Model file for the job. Use its own axes, mm. Face numbers are marked on the shaded views. Round coordinates to 2 decimals unless told otherwise and drop trailing zeros. Write each loop counter-clockwise with the first axis right and the second up, starting at its lowest first coordinate (ties: lowest second). Pieces come first, ordered by that corner, then holes.
```python
from build123d import *

# Parameters (mm, degrees)
BOSS_EXTRUDE1_DEPTH     = 14
SKETCH2_R               = 5
CUT_EXTRUDE1_DEPTH      = 50
SKETCH5_R               = 5
CUT_EXTRUDE3_DEPTH      = 50
CUT_EXTRUDE3_DEPTH_BACK = 50
SKETCH6_R               = 5
CUT_EXTRUDE4_DEPTH      = 50
CUT_EXTRUDE4_DEPTH_BACK = 50


with BuildPart() as part:
    # Sketch1 → Boss-Extrude1 (new body)
    with BuildSketch(Plane.XY):
        Polygon((-42.857142857, 0), (82.142857143, 0), (19.642857143, 108.253175473), align=None)
    extrude(amount=BOSS_EXTRUDE1_DEPTH)

    # Sketch2 → Cut-Extrude1 (cut)
    with BuildSketch(Plane(origin=(0, 0, 0), x_dir=(0, 0, -1), z_dir=(1, 0, 0))):
        with Locations((-7, 101.253175473)):
            Circle(SKETCH2_R)
    extrude(amount=CUT_EXTRUDE1_DEPTH, mode=Mode.SUBTRACT)

    # Sketch5 → Cut-Extrude3 (cut, two sides)
    with BuildSketch(Plane(origin=(-10.714285714, 18.557687224, 0), x_dir=(-0.866025404, -0.5, 0), z_dir=(0.5, -0.866025404, 0))) as cut_extrude3_sk:
        with Locations((30.115374448, -7)):
            Circle(SKETCH5_R)
    extrude(amount=CUT_EXTRUDE3_DEPTH, mode=Mode.SUBTRACT)
    extrude(cut_extrude3_sk.sketch, amount=-CUT_EXTRUDE3_DEPTH_BACK, mode=Mode.SUBTRACT)

    # Sketch6 → Cut-Extrude4 (cut, two sides)
    with BuildSketch(Plane(origin=(20.535714286, 35.568900513, 0), x_dir=(0.866025404, -0.5, 0), z_dir=(0.5, 0.866025404, 0))) as cut_extrude4_sk:
        with Locations((64.137801025, -7)):
            Circle(SKETCH6_R)
    extrude(amount=CUT_EXTRUDE4_DEPTH, mode=Mode.SUBTRACT)
    extrude(cut_extrude4_sk.sketch, amount=-CUT_EXTRUDE4_DEPTH_BACK, mode=Mode.SUBTRACT)


solid = part.part
```
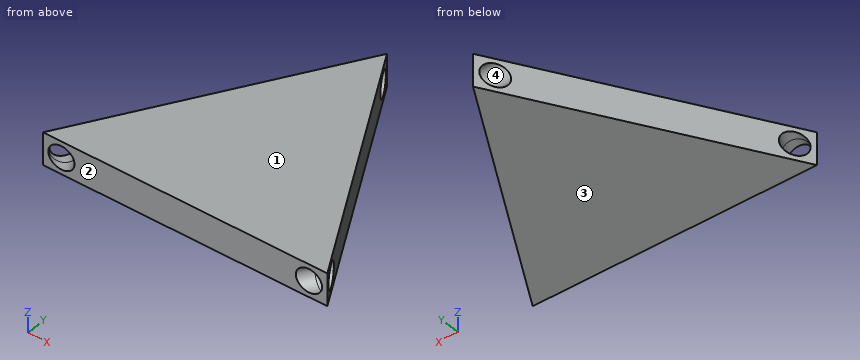
1) Pull direction Z, two halves, no side cores. Call the marked faces 1, 2, 3 and 4: released by +Z, released by -Z, zero draft, split by the parting line, or undercut.
2) Wall check: probe 1 along Y at (x, z) = (20.25, 7); probe 2 along Y at (x, z) = (16, 7); probe 3 along Y at (x, z) = (5, 6). Give the ranges that are in metal, low to high.
3) Cut at C-C on x = 53. List the corners of the cut face in (y, z), and give its area (3 significant figures).
4) Cut at B-B on y = 68. List the corners of the cut face in (x, z), and give its area (3 significant figures).
5) Flat gauge pins, fed straight in: pin 1 Ø1.5 at (y, z) = (86, 5) entering from -X; pin 2 Ø1 at (y, z) = (20, 3) entering from +X; pin 3 Ø12 at (x, y) = (69, 35) entering from -Z; pin 4 Ø8 at (x, y) = (2, 14) entering from -Z. Where does each tip first touch, or does it go through?
6) Cut at A-A on z = 9.25. List the corners of the cut face in (x, y).
Result sheet:
1. face 1: released by +Z
1. face 2: zero draft
1. face 3: released by -Z
1. face 4: undercut
2. probe 1: y = 0 to 96.25, 106.25 to 107.2
2. probe 2: y = 0 to 96.25
2. probe 3: y = 0 to 82.89
3. outline: (0, 0) - (50.48, 0) - (50.48, 14) - (0, 14) - close
3. area: 707 mm2
4. outline: (-3.6, 0) - (42.88, 0) - (42.88, 14) - (-3.6, 14) - close
4. area: 651 mm2
5. pin 1: stops at x = 6.36
5. pin 2: stops at x = 70.88
5. pin 3: passes through
5. pin 4: stops at z = 0
6. outline: (-42.86, 0) - (-39.93, 0) - (-41.39, 2.53) - close; (-36.24, 11.47) - (-29.62, 0) - (68.9, 0) - (75.52, 11.47) - (26.26, 96.79) - (13.02, 96.79) - close; (18.18, 105.72) - (21.11, 105.72) - (19.64, 108.25) - close; (79.22, 0) - (82.14, 0) - (80.68, 2.53) - close
